Check sheet for the drawn part. Datum: minimum x, y, z corner. Units: mm. A direction names the side the tool comes from. Give positions to 0.01 mm unless a question says otherwise; leave off trailing zeros. Write each loop counter-clockwise with the first axis right and the second up, starting at its lowest first coordinate (ties: lowest second). Pieces come first, ordered by that corner, then holes. Notation, with made-up numbers: (-10, -8) - (-3, -8) arc R16 cw to (-3, 11) - close; hole circle Ø6 at (59, -15.75). An arc over 180 degrees is marked (long way). Use a Markdown table: item, result.
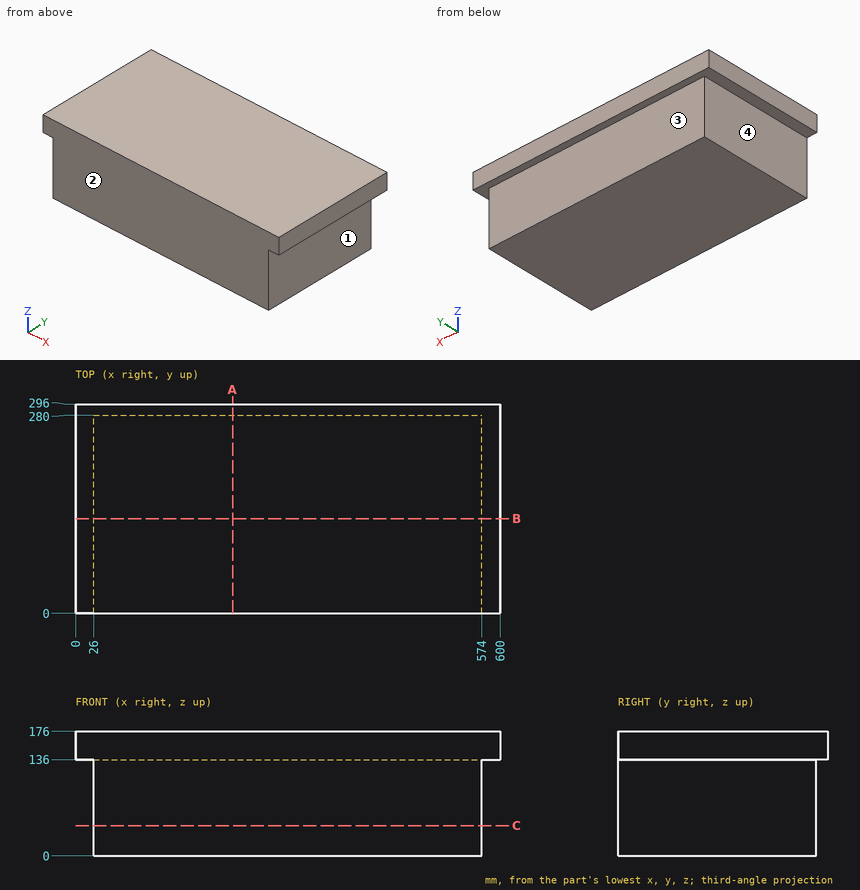
1) Material ranges on L1, parallel to X at y = 249, z = 131; L2, parallel to Y at x = 358, z = 38.5, recorded low to high. Write a range as from..to.
Working result:
| item | result |
|---|---|
| L1 | x = 26..574 |
| L2 | y = 0..280 |
2) Section check C-C on z = 43. Record the boundary of the cut face in (x, y), then the cut area to 3 significant figures.
Working result:
| item | result |
|---|---|
| outline | (26, 0) - (574, 0) - (574, 280) - (26, 280) - close |
| area | 153,000 mm² |
3) Section check A-A on x = 222. Record the boundary of the cut face in (y, z).
Working result:
| item | result |
|---|---|
| outline | (0, 0) - (280, 0) - (280, 136) - (296, 136) - (296, 176) - (0, 176) - close |
4) Depth check by flat-ended pin: P1, Ø3, axis at y = 251, z = 86, coming from the -X side; P2, Ø5, axis at x = 134, z = 76, coming from the +Y side; P3, Ø3, axis at y = 73, z = 31, coming from the +X side. Enter the tip coordinate at first touch or a pass-through.
Working result:
| item | result |
|---|---|
| P1 | stops at x = 26 |
| P2 | stops at y = 280 |
| P3 | stops at x = 574 |
5) Section check B-B on y = 134. Record the boundary of the cut face in (x, z), then the cut area to 3 significant figures.
Working result:
| item | result |
|---|---|
| outline | (0, 136) - (26, 136) - (26, 0) - (574, 0) - (574, 136) - (600, 136) - (600, 176) - (0, 176) - close |
| area | 98,500 mm² |
6) Set-up check for the marked faces 1, 2, 3 and 4: record each of +Z, -Z, +X, -X, +Y, -Y from which the full face is reachable in a straight line by a thin tool's end or side.
Working result:
| item | result |
|---|---|
| face 1 | -Z, +X, +Y, -Y |
| face 2 | +Z, -Z, +X, -X, -Y |
| face 3 | -Z, +X, -X, +Y |
| face 4 | -Z, -X, +Y, -Y |
